Work out the finished part from the listing and answer in its coordinate system (mm). A direction names the side the tool comes from. Coordinates: 2 decimals unless noted, no trailing zeros. Loops run counter-clockwise (first coordinate to the right, second up) from the corner with the lowest first, then second, coordinate; pieces in that order, holes last. Notation, with made-up numbers: M 12,71.5 L 64,71.5 A18 cw 64,86.5 Z; hole C 28.25,83 d9. An arc over 180 degrees is marked long. Write each question's results on one line, items separated by ' | '.
```python
from build123d import *

# Parameters (mm, degrees)
SKETCH1_W           = 56.261
SKETCH1_H           = 56.261
BOSS_EXTRUDE2_DEPTH = 75.4888
SKETCH2_R           = 19.05
BOSS_EXTRUDE3_DEPTH = 1.27
CUT_EXTRUDE1_DEPTH  = 70.3834
FILLET1_R           = 2.54
FILLET2_R           = 1.905
SKETCH4_R           = 2.413
SKETCH4_R_2         = 2.6035
CUT_EXTRUDE2_DEPTH  = 5.1054
BOSS_EXTRUDE4_DEPTH = 20.32
SKETCH6_W           = 11.049
SKETCH6_H           = 11.43
SKETCH6_R           = 2.8575
BOSS_EXTRUDE5_DEPTH = 1.524
SKETCH7_R           = 0.8255
BOSS_EXTRUDE6_DEPTH = 12.7


with BuildPart() as part:
    # Sketch1 → Boss-Extrude2 (new body)
    with BuildSketch(Plane(origin=(0, 0, 0), x_dir=(0, 0, -1), z_dir=(1, 0, 0))):
        Rectangle(SKETCH1_W, SKETCH1_H)
    extrude(amount=BOSS_EXTRUDE2_DEPTH)

    # Sketch2 → Boss-Extrude3 (add)
    with BuildSketch(Plane(origin=(75.4888, 0, 0), x_dir=(0, 0, -1), z_dir=(1, 0, 0))):
        Circle(SKETCH2_R)
    extrude(amount=BOSS_EXTRUDE3_DEPTH)

    # Sketch3 → Cut-Extrude1 (cut)
    with BuildSketch(Plane.ZY):
        with BuildLine():
            Line((28.1305, 18.9865), (24.7015, 18.9865))
            ThreePointArc((24.7015, 18.9865), (20.660384746, 20.660384746), (18.9865, 24.7015))
            Line((18.9865, 24.7015), (18.9865, 28.1305))
            Line((18.9865, 28.1305), (28.1305, 28.1305))
            Line((28.1305, 28.1305), (28.1305, 18.9865))
        make_face()
        with BuildLine():
            Line((-28.1305, 28.1305), (-18.9865, 28.1305))
            Line((-18.9865, 28.1305), (-18.9865, 24.7015))
            ThreePointArc((-18.9865, 24.7015), (-20.660384746, 20.660384746), (-24.7015, 18.9865))
            Line((-24.7015, 18.9865), (-28.1305, 18.9865))
            Line((-28.1305, 18.9865), (-28.1305, 28.1305))
        make_face()
        with BuildLine():
            Line((18.9865, -28.1305), (18.9865, -24.7015))
            ThreePointArc((18.9865, -24.7015), (20.660384746, -20.660384746), (24.7015, -18.9865))
            Line((24.7015, -18.9865), (28.1305, -18.9865))
            Line((28.1305, -18.9865), (28.1305, -28.1305))
            Line((28.1305, -28.1305), (18.9865, -28.1305))
        make_face()
        with BuildLine():
            Line((-28.1305, -18.9865), (-24.7015, -18.9865))
            ThreePointArc((-24.7015, -18.9865), (-20.660384746, -20.660384746), (-18.9865, -24.7015))
            Line((-18.9865, -24.7015), (-18.9865, -28.1305))
            Line((-18.9865, -28.1305), (-28.1305, -28.1305))
            Line((-28.1305, -28.1305), (-28.1305, -18.9865))
        make_face()
    extrude(amount=-CUT_EXTRUDE1_DEPTH, mode=Mode.SUBTRACT)

    # Fillet1
    fillet1_edges = [part.edges().sort_by_distance(p)[0] for p in [
        (72.9361, -28.1305, -28.1305),
        (72.9361, -28.1305, 28.1305),
        (72.9361, 28.1305, 28.1305),
        (72.9361, 28.1305, -28.1305),
    ]]
    fillet(fillet1_edges, radius=FILLET1_R)

    # Fillet2
    fillet2_edges = [part.edges().sort_by_distance(p)[0] for p in [
        (35.1917, -28.1305, -18.9865),
        (35.1917, -18.9865, -28.1305),
        (35.1917, -18.9865, 28.1305),
        (35.1917, -28.1305, 18.9865),
        (35.1917, 28.1305, 18.9865),
        (35.1917, 18.9865, 28.1305),
        (35.1917, 18.9865, -28.1305),
        (35.1917, 28.1305, -18.9865),
    ]]
    fillet(fillet2_edges, radius=FILLET2_R)

    # Sketch4 → Cut-Extrude2 (cut)
    with BuildSketch(Plane.ZY.offset(-70.3834)):
        with Locations((-23.6855, 23.6855)):
            Circle(SKETCH4_R)
        with Locations((23.6855, 23.6855)):
            Circle(SKETCH4_R)
        with Locations((23.6855, -23.6855)):
            Circle(SKETCH4_R_2)
        with Locations((-23.6855, -23.6855)):
            Circle(SKETCH4_R_2)
    extrude(amount=-CUT_EXTRUDE2_DEPTH, mode=Mode.SUBTRACT)

    # Sketch5 → Boss-Extrude4 (add)
    with BuildSketch(Plane(origin=(76.7588, 0, 0), x_dir=(0, 0, -1), z_dir=(1, 0, 0))):
        with BuildLine():
            Line((-2.295189031, 3.2766), (2.295189031, 3.2766))
            ThreePointArc((2.295189031, 3.2766), (0, -4.0005), (-2.295189031, 3.2766))
        make_face()
    extrude(amount=BOSS_EXTRUDE4_DEPTH)

    # Sketch6 → Boss-Extrude5 (add)
    with BuildSketch(Plane.XZ.offset(28.1305)):
        with Locations((5.5245, 0)):
            Rectangle(SKETCH6_W, SKETCH6_H)
        with Locations((6.858, 0)):
            Circle(SKETCH6_R, mode=Mode.SUBTRACT)
    extrude(amount=BOSS_EXTRUDE5_DEPTH)

    # Sketch7 → Boss-Extrude6 (add)
    with BuildSketch(Plane.XZ.offset(28.1305)):
        with Locations((6.858, 1.285488676)):
            Circle(SKETCH7_R)
        with Locations((8.143488676, 0)):
            Circle(SKETCH7_R)
        with Locations((6.858, -1.285488676)):
            Circle(SKETCH7_R)
        with Locations((5.572511324, 0)):
            Circle(SKETCH7_R)
    extrude(amount=BOSS_EXTRUDE6_DEPTH)


solid = part.part
```
1) Find section A-A, the plane y = 22.5. Give the vertices of the cut face in (x, z).
Check result:
outline: M 0,-19.43 L 70.38,-19.43 L 70.38,-21.58 L 75.49,-21.58 L 75.49,21.58 L 70.38,21.58 L 70.38,19.43 L 0,19.43 Z; M 70.38,-28.13 L 75.49,-28.13 L 75.49,-25.79 L 70.38,-25.79 Z; M 70.38,25.79 L 75.49,25.79 L 75.49,28.13 L 70.38,28.13 Z
2) Find section D-D, the plane z = -14. Give the vertices of the cut face in (x, y), and give its area (3 significant figures).
Check result:
outline: M 0,-28.13 L 75.49,-28.13 L 75.49,-12.92 L 76.76,-12.92 L 76.76,12.92 L 75.49,12.92 L 75.49,28.13 L 0,28.13 Z | area: 4,280 mm^2
3) For a pull along Z with two mould halves and no side action, classify faces 5 (the face through (37, 28.13, 0)), 6 (the face through (34.699, -20.705, 20.616)), 7 (the face through (76.11, -11.59, 15.12)), 8 (the face through (72.9, 24.41, 25.987)) as released by +Z, released by -Z, zero draft, split by the parting line, or undercut.
Check result:
face 5: zero draft | face 6: released by +Z | face 7: split by the parting line | face 8: undercut
4) Find section B-B, the plane y = 0. Give the vertices of the cut face in (x, z).
Check result:
outline: M 0,-28.13 L 75.49,-28.13 L 75.49,-19.05 L 76.76,-19.05 L 76.76,-4 L 97.08,-4 L 97.08,4 L 76.76,4 L 76.76,19.05 L 75.49,19.05 L 75.49,28.13 L 0,28.13 Z
5) Straight lines are drawn through the part: probe 1 along X at (y, z) = (-17.5, 19); probe 2 along X at (y, z) = (-6.5, 12.5); probe 3 along Y at (x, z) = (33, -25). For each, find the intervals that lie inside material, in ascending order. Write a range as [from, to].
Check result:
probe 1: [0, 75.49] | probe 2: [0, 76.76] | probe 3: [-18.99, 18.99]
6) Given pin 1 Ø3.5 at (y, z) = (-25, 24.5) entering from -X; pin 2 Ø7.5 at (y, z) = (23.69, -23.69) entering from +X; pin 3 Ø0.5 at (y, z) = (-28.5, -1) entering from +X; pin 4 Ø3 at (y, z) = (-23.69, -23.69) entering from -X, each flat-ended and moving along its own axis, determine where each tip first touches the part or whether it passes through.
Check result:
pin 1: x = 70.38 | pin 2: x = 75.49 | pin 3: x = 11.05 | pin 4: through
7) Which of the six approach directions +Z, -Z, +X, -X, +Y, -Y give full straight-line access (tool end or side, diameter ignored) to faces 1 (the face through (34.699, -20.616, -20.705)), 2 (the face through (75.489, 19, 7)), 3 (the face through (34.699, 20.705, -20.616)), 4 (the face through (7, -28.13, 0))?
Check result:
face 1: -Z, -X, -Y | face 2: +X | face 3: -Z, -X, +Y | face 4: -Y
8) Find section C-C, the plane x = 50.5. Give the vertices of the cut face in (y, z) (1 decimal).
Check result:
outline: M -28.1,-17.1 A1.9 ccw -26.2,-19 L -24.7,-19 A5.7 cw -19,-24.7 L -19,-26.2 A1.9 ccw -17.1,-28.1 L 17.1,-28.1 A1.9 ccw 19,-26.2 L 19,-24.7 A5.7 cw 24.7,-19 L 26.2,-19 A1.9 ccw 28.1,-17.1 L 28.1,17.1 A1.9 ccw 26.2,19 L 24.7,19 A5.7 cw 19,24.7 L 19,26.2 A1.9 ccw 17.1,28.1 L -17.1,28.1 A1.9 ccw -19,26.2 L -19,24.7 A5.7 cw -24.7,19 L -26.2,19 A1.9 ccw -28.1,17.1 Z
